```python
from build123d import *

# Parameters (mm, degrees)
EXTRUDE1_DEPTH          = 22.86
EXTRUDE1_DEPTH_BACK     = 22.86
EXTRUDE3_0_START        = 3.81
SKETCH3_1_OUTSIDE_W     = 30.048
SKETCH3_1_OUTSIDE_H     = 32.75
SKETCH3_1_OUTSIDE_R     = 8.73125
EXTRUDE3_0_DEPTH        = 19.05
EXTRUDE3_1_START        = -3.81
SKETCH3_1_2_OUTSIDE_W   = 30.048
SKETCH3_1_2_OUTSIDE_H   = 32.75
SKETCH3_1_2_OUTSIDE_R   = 8.73125
EXTRUDE3_1_DEPTH        = 19.05
SKETCH3_2_OUTSIDE_W     = 136.808
SKETCH3_2_OUTSIDE_H     = 139.51
SKETCH3_2_OUTSIDE_R     = 8.73125
EXTRUDE3_2_DEPTH        = 30.818952508
EXTRUDE3_2_DRAFT        = -60
SKETCH3_3_OUTSIDE_W     = 136.808
SKETCH3_3_OUTSIDE_H     = 139.51
SKETCH3_3_OUTSIDE_R     = 8.73125
EXTRUDE3_3_DEPTH        = 30.818952508
EXTRUDE3_3_DRAFT        = -60
FILLET1_R               = 0.396875
EXTRUDE3_4_REACH        = 28.492
EXTRUDE3_4_START_RADIUS = 8.73125
EXTRUDE3_4_END_RADIUS   = 8.73125
CIRPATTERN3_COUNT       = 2
EXTRUDE4_DEPTH          = 27.466216775
EXTRUDE4_DEPTH_BACK     = 27.466216775
SKETCH4_R               = 4.6228
EXTRUDE5_DEPTH          = 3.81
EXTRUDE5_DEPTH_BACK     = 3.81
SKETCH5_R               = 4.6228


with BuildPart() as part:
    # Sketch1.1 → Extrude1 (new, two sides: drawn at the far end of the back side and taken through both)
    with BuildSketch(Plane.XY.offset(-EXTRUDE1_DEPTH_BACK)):
        Polygon((0, 10.081979076), (-8.73125, 5.040989538), (-8.73125, -5.040989538), (0, -10.081979076), (8.73125, -5.040989538), (8.73125, 5.040989538), align=None)
    extrude(amount=EXTRUDE1_DEPTH + EXTRUDE1_DEPTH_BACK)

    # Sketch3.1 outside → Extrude3.0 (cut)
    with BuildSketch(Plane.XY.offset(EXTRUDE3_0_START)):
        Rectangle(SKETCH3_1_OUTSIDE_W, SKETCH3_1_OUTSIDE_H)
        Circle(SKETCH3_1_OUTSIDE_R, mode=Mode.SUBTRACT)
    extrude(amount=EXTRUDE3_0_DEPTH, mode=Mode.SUBTRACT)

    # Sketch3.1<2> outside → Extrude3.1 (cut)
    with BuildSketch(Plane.XY.offset(EXTRUDE3_1_START)):
        Rectangle(SKETCH3_1_2_OUTSIDE_W, SKETCH3_1_2_OUTSIDE_H)
        Circle(SKETCH3_1_2_OUTSIDE_R, mode=Mode.SUBTRACT)
    extrude(amount=-EXTRUDE3_1_DEPTH, mode=Mode.SUBTRACT)


with BuildPart() as extrude3_2_tool:
    # Sketch3.2 outside → Extrude3.2 (with draft: the straight prism first)
    with BuildSketch(Plane.XY.offset(3.81)):
        Rectangle(SKETCH3_2_OUTSIDE_W, SKETCH3_2_OUTSIDE_H)
        Circle(SKETCH3_2_OUTSIDE_R, mode=Mode.SUBTRACT)
    extrude(amount=-EXTRUDE3_2_DEPTH)
    # Extrude3.2: the draft: its side faces are tilted about the plane it starts from
    extrude3_2_sides = [extrude3_2_tool.faces().sort_by_distance(p)[0] for p in [
        (0, -69.755, -11.599476254),
        (68.404, 0, -11.599476254),
        (0, 69.755, -11.599476254),
        (-68.404, 0, -11.599476254),
        (-8.73125, 0, -11.599476254),
    ]]
    draft(extrude3_2_sides, Plane.XY.offset(3.81), EXTRUDE3_2_DRAFT)


with BuildPart() as part_1:
    add(part.part)

    # Extrude3.2: cut by extrude3_2_tool
    add(extrude3_2_tool.part, mode=Mode.SUBTRACT)


with BuildPart() as extrude3_3_tool:
    # Sketch3.3 outside → Extrude3.3 (with draft: the straight prism first)
    with BuildSketch(Plane(origin=(0, 0, -3.81), x_dir=(-1, 0, 0), z_dir=(0, 0, -1))):
        Rectangle(SKETCH3_3_OUTSIDE_W, SKETCH3_3_OUTSIDE_H)
        with Locations(Location((0, 0, 0), (0, 0, 180))):
            Circle(SKETCH3_3_OUTSIDE_R, mode=Mode.SUBTRACT)
    extrude(amount=-EXTRUDE3_3_DEPTH)
    # Extrude3.3: the draft: its side faces are tilted about the plane it starts from
    extrude3_3_sides = [extrude3_3_tool.faces().sort_by_distance(p)[0] for p in [
        (0, -69.755, 11.599476254),
        (-68.404, 0, 11.599476254),
        (0, 69.755, 11.599476254),
        (68.404, 0, 11.599476254),
        (-8.73125, 0, 11.599476254),
    ]]
    draft(extrude3_3_sides, Plane(origin=(0, 0, -3.81), x_dir=(-1, 0, 0), z_dir=(0, 0, -1)), EXTRUDE3_3_DRAFT)


with BuildPart() as part_2:
    add(part_1.part)

    # Extrude3.3: cut by extrude3_3_tool
    add(extrude3_3_tool.part, mode=Mode.SUBTRACT)

    # Fillet1
    fillet1_edges = [part_2.edges().sort_by_distance(p)[0] for p in [
        (-8.73125, 0, 22.86),
        (-8.73125, 0, -22.86),
    ]]
    fillet(fillet1_edges, radius=FILLET1_R)

    # Extrude3.4: from a cylinder face, 28.492 long prism both ways, kept between that surface and its translate by the depth
    extrude3_4_start = Plane(origin=(0, 0, -13.414881), z_dir=(0, 0, 1)) * Cylinder(EXTRUDE3_4_START_RADIUS, 75.4465, mode=Mode.PRIVATE)
    extrude3_4_end = Plane(origin=(-0.0254, 0, -13.414881), z_dir=(0, 0, 1)) * Cylinder(EXTRUDE3_4_END_RADIUS, 75.4465, mode=Mode.PRIVATE)
    # Sketch3.4 → Extrude3.4 (cut, from a surface)
    with BuildSketch(Plane(origin=(0, 0, 0), x_dir=(0, 0, -1), z_dir=(1, 0, 0)), mode=Mode.PRIVATE) as extrude3_4_sk1:
        Polygon((10.16, 1.5875), (11.5490625, 0.1984375), (15.840639961, 0.1984375), (14.9225, 1.338579148), (15.231608679, 1.5875), (16.51, 0), (14.9225, -1.5875), (14.673579148, -1.338579148), (15.813720797, -0.1984375), (11.5490625, -0.1984375), (10.16, -1.5875), (9.911079148, -1.338579148), (11.249658297, 0), (9.911079148, 1.338579148), align=None)
    extrude3_4_tool1 = extrude(extrude3_4_sk1.sketch, amount=EXTRUDE3_4_REACH, both=True, mode=Mode.PRIVATE)
    extrude3_4 = ((extrude3_4_tool1 & extrude3_4_start) - extrude3_4_end).solids().sort_by_distance((8.645784, 0.002778, -13.414881))[0]
    add(extrude3_4, mode=Mode.SUBTRACT)

    # CirPattern3: Extrude3.4 ×2 about axis
    cirpattern3_axis = Axis((0, 0, 0), (0, 0, 1))
    for i in range(1, CIRPATTERN3_COUNT):
        add(extrude3_4.rotate(cirpattern3_axis, i * 360 / CIRPATTERN3_COUNT), mode=Mode.SUBTRACT)

    # Sketch4 → Extrude4 (cut, two sides: drawn at the far end of the back side and taken through both)
    with BuildSketch(Plane.XY.offset(-EXTRUDE4_DEPTH_BACK)):
        Circle(SKETCH4_R)
    extrude(amount=EXTRUDE4_DEPTH + EXTRUDE4_DEPTH_BACK, mode=Mode.SUBTRACT)

    # Sketch5 → Extrude5 (add, two sides: drawn at the far end of the back side and taken through both)
    with BuildSketch(Plane.XY.offset(-EXTRUDE5_DEPTH_BACK)):
        Circle(SKETCH5_R)
    extrude(amount=EXTRUDE5_DEPTH + EXTRUDE5_DEPTH_BACK)


solid = part_2.part
```
Source: CAD feature listing. Evaluate the final solid. Frame: model axes, mm. A direction names the side the tool comes from. Give positions to 0.01 mm unless a question says otherwise; leave off trailing zeros. Write each loop counter-clockwise with the first axis right and the second up, starting at its lowest first coordinate (ties: lowest second). Pieces come first, ordered by that corner, then holes.
1. Material intervals for line 1 along Y through (x, z) = (0, -11.5); line 2 along Y through (x, z) = (1.5, 8.5), sorted ascending.
2. Access query for faces 1 (the face through (7.9, 4.5, 3.6)), 2 (the face through (-3.67, -2.81, -13.47)). Directions: +Z, -Z, +X, -X, +Y, -Y. A direction counts if a zero-diameter tool reaches every point of the face in a straight line with its end or side. Return the directions, or none.
3. Section query B-B (z = 0). Return the cut outline in (x, y), then the cut area to 3 significant figures.
4. Section query A-A (z = 16.5). Return the cut outline in (x, y).
5. First-contact query: pin 1 (5 mm diameter, centred on y = 3, z = 8.5, fed in from -X); pin 2 (3 mm diameter, centred on x = -6, z = 0.5, fed in from -Y); pin 3 (10 mm diameter, centred on x = 1.5, y = -1, fed in from +Z); pin 4 (7.5 mm diameter, centred on x = 0, y = 0, fed in from -Z). Flat tips, straight axial feed; report the tip coordinate or a pass-through.
6. Pull-direction query (Y, two-part tool) for faces 3 (the face through (4, -4, 22.86)), 4 (the face through (0, 0, 3.81)), 5 (the face through (-6.93, -5.31, 13.01)); classes: +Y half, -Y half, draft (parallel to the pull), parting line (faces both ways), or undercut.
Output values:
1. line 1: y = -8.73 to -4.62, 4.62 to 8.73
1. line 2: y = -8.6 to -4.37, 4.37 to 8.6
2. face 1: +Z, +X, +Y
2. face 2: -Z
3. outline: (-8.73, -5.04) - (0, -10.08) - (8.73, -5.04) - (8.73, 5.04) - (0, 10.08) - (-8.73, 5.04) - close
3. area: 264 mm2
4. outline: circle Ø17.46 at (0, 0); hole circle Ø9.25 at (0, 0)
5. pin 1: stops at x = -8.72
5. pin 2: stops at y = -7.48
5. pin 3: stops at z = 22.86
5. pin 4: stops at z = -3.81
6. face 3: draft
6. face 4: undercut
6. face 5: parting line
